Check sheet for the modelled part. Datum: model origin and axes. Units: mm. A direction names the side the tool comes from. Round coordinates to 2 decimals unless told otherwise and drop trailing zeros. Write each loop counter-clockwise with the first axis right and the second up, starting at its lowest first coordinate (ties: lowest second). Pieces come first, ordered by that corner, then holes. Notation, with made-up numbers: (67.25, 58.25) -> (126.25, 58.25) arc R30 ccw to (126.25, 87.25) -> close; hole circle Ø10 at (76.25, 29). An arc over 180 degrees is marked (long way). Write item = value, one per line.
from build123d import *

# Parameters (mm, degrees)
F0_R     = 1.05
F0_R_2   = 1
F1_DEPTH = 0.6
F2_DEPTH = 1


with BuildPart() as f1:
    # F0 (on Top) → F1 (new body)
    with BuildSketch(Plane.XY):
        with BuildLine():
            Line((-10.25, -11.35), (10.25, -11.35))
            ThreePointArc((10.25, -11.35), (11.487437, -10.837437), (12, -9.6))
            Line((12, -9.6), (12, 11.35))
            Line((12, 11.35), (13, 11.35))
            Line((13, 11.35), (13, 12.65))
            Line((13, 12.65), (1.4, 12.65))
            ThreePointArc((1.4, 12.65), (1.117157, 12.767157), (1, 13.05))
            Line((1, 13.05), (1, 14.65))
            Line((1, 14.65), (1.6, 14.65))
            ThreePointArc((1.6, 14.65), (1.882843, 14.767157), (2, 15.05))
            Line((2, 15.05), (2, 18.25))
            ThreePointArc((2, 18.25), (1.882843, 18.532843), (1.6, 18.65))
            Line((1.6, 18.65), (-1.6, 18.65))
            ThreePointArc((-1.6, 18.65), (-1.882843, 18.532843), (-2, 18.25))
            Line((-2, 18.25), (-2, 15.05))
            ThreePointArc((-2, 15.05), (-1.882843, 14.767157), (-1.6, 14.65))
            Line((-1.6, 14.65), (-1, 14.65))
            Line((-1, 14.65), (-1, 13.05))
            ThreePointArc((-1, 13.05), (-1.117157, 12.767157), (-1.4, 12.65))
            Line((-1.4, 12.65), (-13, 12.65))
            Line((-13, 12.65), (-13, 11.35))
            Line((-13, 11.35), (-12, 11.35))
            Line((-12, 11.35), (-12, -9.6))
            ThreePointArc((-12, -9.6), (-11.487437, -10.837437), (-10.25, -11.35))
        make_face()
        with BuildLine():
            ThreePointArc((-5, 2.25), (-4.853553, 2.603553), (-4.5, 2.75))
            Line((-4.5, 2.75), (-4.5, 3.374709))
            ThreePointArc((-4.5, 3.374709), (-4.353553, 3.728262), (-4, 3.874709))
            Line((-4, 3.874709), (-3.5, 3.874709))
            ThreePointArc((-3.5, 3.874709), (-3.146447, 3.728262), (-3, 3.374709))
            Line((-3, 3.374709), (-3, 2.75))
            Line((-3, 2.75), (-0.75, 2.75))
            Line((-0.75, 2.75), (-0.75, 3.374709))
            ThreePointArc((-0.75, 3.374709), (-0.603553, 3.728262), (-0.25, 3.874709))
            Line((-0.25, 3.874709), (0.25, 3.874709))
            ThreePointArc((0.25, 3.874709), (0.603553, 3.728262), (0.75, 3.374709))
            Line((0.75, 3.374709), (0.75, 2.75))
            Line((0.75, 2.75), (3, 2.75))
            Line((3, 2.75), (3, 3.374709))
            ThreePointArc((3, 3.374709), (3.146447, 3.728262), (3.5, 3.874709))
            Line((3.5, 3.874709), (4, 3.874709))
            ThreePointArc((4, 3.874709), (4.353553, 3.728262), (4.5, 3.374709))
            Line((4.5, 3.374709), (4.5, 2.75))
            ThreePointArc((4.5, 2.75), (4.853553, 2.603553), (5, 2.25))
            Line((5, 2.25), (5, -4.95))
            ThreePointArc((5, -4.95), (4.853553, -5.303553), (4.5, -5.45))
            Line((4.5, -5.45), (4.5, -6.225291))
            ThreePointArc((4.5, -6.225291), (4.353553, -6.578845), (4, -6.725291))
            Line((4, -6.725291), (3.5, -6.725291))
            ThreePointArc((3.5, -6.725291), (3.146447, -6.578845), (3, -6.225291))
            Line((3, -6.225291), (3, -5.45))
            Line((3, -5.45), (0.75, -5.45))
            Line((0.75, -5.45), (0.75, -6.225291))
            ThreePointArc((0.75, -6.225291), (0.603553, -6.578845), (0.25, -6.725291))
            Line((0.25, -6.725291), (-0.25, -6.725291))
            ThreePointArc((-0.25, -6.725291), (-0.603553, -6.578845), (-0.75, -6.225291))
            Line((-0.75, -6.225291), (-0.75, -5.45))
            Line((-0.75, -5.45), (-3, -5.45))
            Line((-3, -5.45), (-3, -6.225291))
            ThreePointArc((-3, -6.225291), (-3.146447, -6.578845), (-3.5, -6.725291))
            Line((-3.5, -6.725291), (-4, -6.725291))
            ThreePointArc((-4, -6.725291), (-4.353553, -6.578845), (-4.5, -6.225291))
            Line((-4.5, -6.225291), (-4.5, -5.45))
            ThreePointArc((-4.5, -5.45), (-4.853553, -5.303553), (-5, -4.95))
            Line((-5, -4.95), (-5, 2.25))
        make_face(mode=Mode.SUBTRACT)
        with Locations((-8.75, 10.65)):
            Circle(F0_R, mode=Mode.SUBTRACT)
        with Locations((8.75, 10.65)):
            Circle(F0_R, mode=Mode.SUBTRACT)
        with Locations((0, 16.65)):
            Circle(F0_R_2, mode=Mode.SUBTRACT)
        with BuildLine():
            Line((-4.5, 3.374709), (-4.5, 2.75))
            Line((-4.5, 2.75), (-3, 2.75))
            Line((-3, 2.75), (-3, 3.374709))
            ThreePointArc((-3, 3.374709), (-3.146447, 3.728262), (-3.5, 3.874709))
            Line((-3.5, 3.874709), (-4, 3.874709))
            ThreePointArc((-4, 3.874709), (-4.353553, 3.728262), (-4.5, 3.374709))
        make_face()
        with BuildLine():
            Line((-0.75, 3.374709), (-0.75, 2.75))
            Line((-0.75, 2.75), (0.75, 2.75))
            Line((0.75, 2.75), (0.75, 3.374709))
            ThreePointArc((0.75, 3.374709), (0.603553, 3.728262), (0.25, 3.874709))
            Line((0.25, 3.874709), (-0.25, 3.874709))
            ThreePointArc((-0.25, 3.874709), (-0.603553, 3.728262), (-0.75, 3.374709))
        make_face()
        with BuildLine():
            Line((3, 3.374709), (3, 2.75))
            Line((3, 2.75), (4.5, 2.75))
            Line((4.5, 2.75), (4.5, 3.374709))
            ThreePointArc((4.5, 3.374709), (4.353553, 3.728262), (4, 3.874709))
            Line((4, 3.874709), (3.5, 3.874709))
            ThreePointArc((3.5, 3.874709), (3.146447, 3.728262), (3, 3.374709))
        make_face()
        with BuildLine():
            Line((4.5, -5.45), (3, -5.45))
            Line((3, -5.45), (3, -6.225291))
            ThreePointArc((3, -6.225291), (3.146447, -6.578845), (3.5, -6.725291))
            Line((3.5, -6.725291), (4, -6.725291))
            ThreePointArc((4, -6.725291), (4.353553, -6.578845), (4.5, -6.225291))
            Line((4.5, -6.225291), (4.5, -5.45))
        make_face()
        with BuildLine():
            Line((0.75, -5.45), (-0.75, -5.45))
            Line((-0.75, -5.45), (-0.75, -6.225291))
            ThreePointArc((-0.75, -6.225291), (-0.603553, -6.578845), (-0.25, -6.725291))
            Line((-0.25, -6.725291), (0.25, -6.725291))
            ThreePointArc((0.25, -6.725291), (0.603553, -6.578845), (0.75, -6.225291))
            Line((0.75, -6.225291), (0.75, -5.45))
        make_face()
        with BuildLine():
            Line((-3, -5.45), (-4.5, -5.45))
            Line((-4.5, -5.45), (-4.5, -6.225291))
            ThreePointArc((-4.5, -6.225291), (-4.353553, -6.578845), (-4, -6.725291))
            Line((-4, -6.725291), (-3.5, -6.725291))
            ThreePointArc((-3.5, -6.725291), (-3.146447, -6.578845), (-3, -6.225291))
            Line((-3, -6.225291), (-3, -5.45))
        make_face()
    extrude(amount=F1_DEPTH)

    # F0 (on Top) → F2 (join)
    with BuildSketch(Plane.XY):
        with BuildLine():
            Line((-10.25, -11.35), (10.25, -11.35))
            ThreePointArc((10.25, -11.35), (11.487437, -10.837437), (12, -9.6))
            Line((12, -9.6), (12, 11.35))
            Line((12, 11.35), (13, 11.35))
            Line((13, 11.35), (13, 12.65))
            Line((13, 12.65), (1.4, 12.65))
            ThreePointArc((1.4, 12.65), (1.117157, 12.767157), (1, 13.05))
            Line((1, 13.05), (1, 14.65))
            Line((1, 14.65), (1.6, 14.65))
            ThreePointArc((1.6, 14.65), (1.882843, 14.767157), (2, 15.05))
            Line((2, 15.05), (2, 18.25))
            ThreePointArc((2, 18.25), (1.882843, 18.532843), (1.6, 18.65))
            Line((1.6, 18.65), (-1.6, 18.65))
            ThreePointArc((-1.6, 18.65), (-1.882843, 18.532843), (-2, 18.25))
            Line((-2, 18.25), (-2, 15.05))
            ThreePointArc((-2, 15.05), (-1.882843, 14.767157), (-1.6, 14.65))
            Line((-1.6, 14.65), (-1, 14.65))
            Line((-1, 14.65), (-1, 13.05))
            ThreePointArc((-1, 13.05), (-1.117157, 12.767157), (-1.4, 12.65))
            Line((-1.4, 12.65), (-13, 12.65))
            Line((-13, 12.65), (-13, 11.35))
            Line((-13, 11.35), (-12, 11.35))
            Line((-12, 11.35), (-12, -9.6))
            ThreePointArc((-12, -9.6), (-11.487437, -10.837437), (-10.25, -11.35))
        make_face()
        with BuildLine():
            ThreePointArc((-5, 2.25), (-4.853553, 2.603553), (-4.5, 2.75))
            Line((-4.5, 2.75), (-4.5, 3.374709))
            ThreePointArc((-4.5, 3.374709), (-4.353553, 3.728262), (-4, 3.874709))
            Line((-4, 3.874709), (-3.5, 3.874709))
            ThreePointArc((-3.5, 3.874709), (-3.146447, 3.728262), (-3, 3.374709))
            Line((-3, 3.374709), (-3, 2.75))
            Line((-3, 2.75), (-0.75, 2.75))
            Line((-0.75, 2.75), (-0.75, 3.374709))
            ThreePointArc((-0.75, 3.374709), (-0.603553, 3.728262), (-0.25, 3.874709))
            Line((-0.25, 3.874709), (0.25, 3.874709))
            ThreePointArc((0.25, 3.874709), (0.603553, 3.728262), (0.75, 3.374709))
            Line((0.75, 3.374709), (0.75, 2.75))
            Line((0.75, 2.75), (3, 2.75))
            Line((3, 2.75), (3, 3.374709))
            ThreePointArc((3, 3.374709), (3.146447, 3.728262), (3.5, 3.874709))
            Line((3.5, 3.874709), (4, 3.874709))
            ThreePointArc((4, 3.874709), (4.353553, 3.728262), (4.5, 3.374709))
            Line((4.5, 3.374709), (4.5, 2.75))
            ThreePointArc((4.5, 2.75), (4.853553, 2.603553), (5, 2.25))
            Line((5, 2.25), (5, -4.95))
            ThreePointArc((5, -4.95), (4.853553, -5.303553), (4.5, -5.45))
            Line((4.5, -5.45), (4.5, -6.225291))
            ThreePointArc((4.5, -6.225291), (4.353553, -6.578845), (4, -6.725291))
            Line((4, -6.725291), (3.5, -6.725291))
            ThreePointArc((3.5, -6.725291), (3.146447, -6.578845), (3, -6.225291))
            Line((3, -6.225291), (3, -5.45))
            Line((3, -5.45), (0.75, -5.45))
            Line((0.75, -5.45), (0.75, -6.225291))
            ThreePointArc((0.75, -6.225291), (0.603553, -6.578845), (0.25, -6.725291))
            Line((0.25, -6.725291), (-0.25, -6.725291))
            ThreePointArc((-0.25, -6.725291), (-0.603553, -6.578845), (-0.75, -6.225291))
            Line((-0.75, -6.225291), (-0.75, -5.45))
            Line((-0.75, -5.45), (-3, -5.45))
            Line((-3, -5.45), (-3, -6.225291))
            ThreePointArc((-3, -6.225291), (-3.146447, -6.578845), (-3.5, -6.725291))
            Line((-3.5, -6.725291), (-4, -6.725291))
            ThreePointArc((-4, -6.725291), (-4.353553, -6.578845), (-4.5, -6.225291))
            Line((-4.5, -6.225291), (-4.5, -5.45))
            ThreePointArc((-4.5, -5.45), (-4.853553, -5.303553), (-5, -4.95))
            Line((-5, -4.95), (-5, 2.25))
        make_face(mode=Mode.SUBTRACT)
        with Locations((-8.75, 10.65)):
            Circle(F0_R, mode=Mode.SUBTRACT)
        with Locations((8.75, 10.65)):
            Circle(F0_R, mode=Mode.SUBTRACT)
        with Locations((0, 16.65)):
            Circle(F0_R_2, mode=Mode.SUBTRACT)
    extrude(amount=F2_DEPTH)


solid = f1.part
(1) Sectioned sample at B-B on y = 10. Enter the section's corners in (x, z), then the cut area to 3 significant figures.
Worked answers:
outline = (-12, 0) -> (-9.57, 0) -> (-9.57, 1) -> (-12, 1) -> close; (-7.93, 0) -> (7.93, 0) -> (7.93, 1) -> (-7.93, 1) -> close; (9.57, 0) -> (12, 0) -> (12, 1) -> (9.57, 1) -> close
area = 20.7 mm²
(2) Sectioned sample at C-C on y = 0. Enter the section's corners in (x, z).
Worked answers:
outline = (-12, 0) -> (-5, 0) -> (-5, 1) -> (-12, 1) -> close; (5, 0) -> (12, 0) -> (12, 1) -> (5, 1) -> close
(3) Material ranges on L1, parallel to Y at x = -8.75, z = 0.6; L2, parallel to Y at x = -4, z = 0.85; L3, parallel to Y at x = 1.75, z = 0.9, recorded low to high. Write a range as [from, to].
Worked answers:
L1 = [-11.35, 9.6], [11.7, 12.65]
L2 = [-11.35, -6.73], [3.87, 12.65]
L3 = [-11.35, -5.45], [2.75, 12.65], [14.68, 18.62]
(4) Sectioned sample at A-A on x = -8.75. Enter the section's corners in (y, z), then the cut area to 3 significant figures.
Worked answers:
outline = (-11.35, 0) -> (9.6, 0) -> (9.6, 1) -> (-11.35, 1) -> close; (11.7, 0) -> (12.65, 0) -> (12.65, 1) -> (11.7, 1) -> close
area = 21.9 mm²
(5) Sectioned sample at D-D on z = 0.35. Count the separate pieces of the cut face and the enclosed holes in it, then the cut area to 3 significant figures.
Worked answers:
separate_pieces = 1
enclosed_holes = 4
area = 505 mm²
(6) Release check for a two-part mould opening along X. For faces 4 (the flat face through (0, 18.65, 0.5)), 5 (the cylindrical face through (-0.13, 17.64, 0.49)), 6 (the cylindrical face through (11.474, -10.851, 0.493)) record: pulls with the +X half, pulls with the -X half, needs draft (parallel to the pull), parting line crosses it, or undercut.
Worked answers:
face_4 = needs draft
face_5 = undercut
face_6 = pulls with the +X half
(7) Access from +Z, -Z, +X, -X, +Y, -Y to the whole of each face (thin tool, end or side, straight path). Record for faces 1 (the flat face through (4, -6, 0.6)), 2 (the flat face through (0.1, -5.45, 0.4)), 3 (the flat face through (-12, 1, 0.5)).
Worked answers:
face_1 = +Z
face_2 = +Z, -Z
face_3 = +Z, -Z, -X, -Y
